```python
from build123d import *

# Parameters (mm, degrees)
SKETCH1_R           = 3.175
BOSS_EXTRUDE1_DEPTH = 1.5875
FILLET1_R           = 0.79375
CHAMFER1_SIZE       = 0.254


with BuildPart() as part:
    # Sketch1 → Boss-Extrude1 (new body, symmetric)
    with BuildSketch(Plane(origin=(0, 0, 0), x_dir=(1, 0, 0), z_dir=(0, 1, 0))):
        Polygon((2.749630657, 4.7625), (-2.749630657, 4.7625), (-5.499261314, 0), (-2.749630657, -4.7625), (2.749630657, -4.7625), (5.499261314, 0), align=None)
        Circle(SKETCH1_R, mode=Mode.SUBTRACT)
    extrude(amount=BOSS_EXTRUDE1_DEPTH, both=True)

    # Fillet1
    fillet1_edges = [part.edges().sort_by_distance(p)[0] for p in [
        (5.499261314, 0, 0),
        (2.749630657, 0, 4.7625),
        (-2.749630657, 0, 4.7625),
        (-5.499261314, 0, 0),
        (-2.749630657, 0, -4.7625),
        (2.749630657, 0, -4.7625),
    ]]
    fillet(fillet1_edges, radius=FILLET1_R)

    # Chamfer1
    chamfer1_edges = [part.edges().sort_by_distance(p)[0] for p in [
        (-3.175, -1.5875, 0),
        (-3.175, 1.5875, 0),
        (-4.124445986, -1.5875, 2.38125),
        (-4.124445986, 1.5875, 2.38125),
        (4.124445986, -1.5875, -2.38125),
        (4.124445986, -1.5875, 2.38125),
        (0, -1.5875, 4.7625),
        (-4.124445986, -1.5875, -2.38125),
        (0, -1.5875, -4.7625),
        (2.688233881, -1.5875, 4.656157664),
        (-2.688233881, -1.5875, 4.656157664),
        (5.376467762, -1.5875, 0),
        (2.688233881, -1.5875, -4.656157664),
        (-2.688233881, -1.5875, -4.656157664),
        (-5.376467762, -1.5875, 0),
        (-4.124445986, 1.5875, -2.38125),
        (4.124445986, 1.5875, -2.38125),
        (0, 1.5875, -4.7625),
        (0, 1.5875, 4.7625),
        (4.124445986, 1.5875, 2.38125),
        (2.688233881, 1.5875, 4.656157664),
        (-2.688233881, 1.5875, 4.656157664),
        (5.376467762, 1.5875, 0),
        (2.688233881, 1.5875, -4.656157664),
        (-2.688233881, 1.5875, -4.656157664),
        (-5.376467762, 1.5875, 0),
    ]]
    chamfer(chamfer1_edges, length=CHAMFER1_SIZE)


solid = part.part
```
CAD build for the part. Positions are in the model's coordinates, mm. Round coordinates to 2 decimals unless told otherwise and drop trailing zeros. Order: outer loops, then holes, each group sorted by start corner. A loop starts at its lowest first (then second) coordinate and runs counter-clockwise, first axis right, second up. Notation, with made-up numbers: (-35, 29) -> (-24, 29) arc R4 cw to (-24, 34) -> close; hole circle Ø9 at (45, 77). An arc over 180 degrees is marked (long way). Write item = value, one per line.
(1) Drill centre lines: L1, parallel to X at y = 0.1, z = 0 (3 decimals); L2, parallel to Z at x = 0, y = 0.65 (1 decimal); L3, parallel to X at y = -0.65, z = 0.5. Where is each one in solid material? Low to high.
Answers follow:
L1 = -5.376 to -3.175, 3.175 to 5.376
L2 = -4.8 to -3.2, 3.2 to 4.8
L3 = -5.21 to -3.14, 3.14 to 5.21
(2) Flat gauge pin, fed straight in: P1, Ø1, axis at y = -0.5, z = -1.5, coming from the +X side. Where does the tip first touch, or does it go through?
Answers follow:
P1 = 4.92
(3) Pull direction X, two halves, no side cores. Call faces 1 (the flat face through (4.11, 0.02, 2.41)), 2 (the flat face through (0, 0, 4.762)), 3 (the cylindrical face through (-0.69, -0.02, 3.1)): +X half, -X half, draft (parallel to the pull), parting line (faces both ways), or undercut.
Answers follow:
face_1 = +X half
face_2 = draft
face_3 = undercut
(4) Cut at D-D (x = 4.5). Write the cut outline in (y, z).
Answers follow:
outline = (-1.59, -1.22) -> (-1.33, -1.73) -> (1.33, -1.73) -> (1.59, -1.22) -> (1.59, 1.22) -> (1.33, 1.73) -> (-1.33, 1.73) -> (-1.59, 1.22) -> close
